Verification items for the finished model (mm, model axes). A direction names the side the tool comes from. Coordinates: 2 decimals unless noted, no trailing zeros. Loops run counter-clockwise (first coordinate to the right, second up) from the corner with the lowest first, then second, coordinate; pieces in that order, holes last.
Q1. Material ranges on probe 1 along X at (y, z) = (8.75, -109); probe 2 along X at (y, z) = (8, -123.5); probe 3 along Z at (x, y) = (214.5, 4.75), recorded low to high.
Q2. Sectioned sample at A-A (z = -204). Enter the section's corners in (x, y), then the cut area to 3 significant figures.
Q3. Mould release check, pull along Z, two halves, no side actions. Record for faces 4 (the face through (260, 5, -222)), 5 (the face through (-5, 5, -130)), 6 (the face through (-5, 5, -190)): +Z half, -Z half, draft (parallel to the pull), parting line (faces both ways), or undercut.
Q4. Access from +Z, -Z, +X, -X, +Y, -Y to the whole of each face (thin tool, end or side, straight path). Record for faces 1 (the face through (-5, 5, -150)), 2 (the face through (243, 5, -110)), 3 (the face through (0, 5, -120)).
Q5. Sectioned sample at B-B (x = 169). Enter the section's corners in (y, z), then the cut area to 3 significant figures.
Q6. Go/stop test with flat-tipped pins: P1, Ø5, axis at y = 7.5, z = -106, coming from the -X side; P2, Ø3, axis at x = 82, y = 2.5, coming from the +Z side; P3, Ø3, axis at x = 256, y = 7.5, coming from the +Z side. Record where each tip stops, or that it passes through.
```python
from build123d import *

# Parameters (mm, degrees)
F1_DEPTH = 10


# Not quite as in the source:
# - a feature names something its author has since deleted; it is built from what else it names


with BuildPart() as f1:
    # F0 (on Front) → F1 (new body)
    with BuildSketch(Plane.XZ):
        Polygon((135, -100), (135, -110), (115, -110), (115, -100), (95, -100), (95, -110), (75, -110), (75, -100), (55, -100), (55, -110), (35, -110), (35, -100), (15, -100), (15, -110), (0, -110), (0, -130), (-10, -130), (-10, -150), (0, -150), (0, -170), (-10, -170), (-10, -190), (0, -190), (0, -210), (-10, -210), (-10, -234.2857142857), (260, -234.2857142857), (260, -210), (250, -210), (250, -190), (260, -190), (260, -170), (250, -170), (250, -150), (260, -150), (260, -130), (250, -130), (250, -110), (235, -110), (235, -100), (215, -100), (215, -110), (195, -110), (195, -100), (175, -100), (175, -110), (155, -110), (155, -100), align=None)
    extrude(amount=-F1_DEPTH)


solid = f1.part
```
Geometry check:
1. probe 1: x = 15 to 35, 55 to 75, 95 to 115, 135 to 155, 175 to 195, 215 to 235
1. probe 2: x = 0 to 250
1. probe 3: z = -234.29 to -110
2. outline: (0, 0) - (250, 0) - (250, 10) - (0, 10) - close
2. area: 2,500 mm2
3. face 4: draft
3. face 5: +Z half
3. face 6: undercut
4. face 1: -X, +Y, -Y
4. face 2: +Z, +X, +Y, -Y
4. face 3: +Z, -X, +Y, -Y
5. outline: (0, -234.29) - (10, -234.29) - (10, -110) - (0, -110) - close
5. area: 1,240 mm2
6. P1: stops at x = 15
6. P2: stops at z = -110
6. P3: stops at z = -130
